```python
from build123d import *

# Parameters (mm, degrees)
SKETCH2_R          = 1.35
CUT_EXTRUDE1_DEPTH = 64.835726674
SKETCH4_R          = 25
CUT_EXTRUDE2_DEPTH = 64.835726674


with BuildPart() as part:
    # Sketch1 → Revolve1 (revolve)
    with BuildSketch(Plane.XY, mode=Mode.PRIVATE) as revolve1_sk:
        with BuildLine():
            Line((-42.5, 0), (0, 0))
            Line((0, 0), (0, 5))
            Line((0, 5), (-45, 5))
            Line((-45, 5), (-45, 2.5))
            ThreePointArc((-45, 2.5), (-43.232233047, 1.767766953), (-42.5, 0))
        make_face()
    revolve(revolve1_sk.sketch.rotate(Axis((0, 0, 0), (0, 1, 0)), 270), axis=Axis((0, 0, 0), (0, 1, 0)))

    # Sketch2 → Cut-Extrude1 (cut, through all)
    with BuildSketch(Plane(origin=(0, 5, 0), x_dir=(1, 0, 0), z_dir=(0, 1, 0))):
        with Locations(Location((0, 32.5, 0), (0, 0, 270))):
            Circle(SKETCH2_R)
        with Locations(Location((22.980970389, 22.980970389, 0), (0, 0, 270))):
            Circle(SKETCH2_R)
        with Locations(Location((32.5, 0, 0), (0, 0, 270))):
            Circle(SKETCH2_R)
        with Locations(Location((22.980970389, -22.980970389, 0), (0, 0, 270))):
            Circle(SKETCH2_R)
        with Locations(Location((0, -32.5, 0), (0, 0, 270))):
            Circle(SKETCH2_R)
        with Locations(Location((-22.980970389, -22.980970389, 0), (0, 0, 270))):
            Circle(SKETCH2_R)
        with Locations(Location((-32.5, 0, 0), (0, 0, 270))):
            Circle(SKETCH2_R)
        with Locations(Location((-22.980970389, 22.980970389, 0), (0, 0, 270))):
            Circle(SKETCH2_R)
    extrude(amount=-CUT_EXTRUDE1_DEPTH, mode=Mode.SUBTRACT)

    # Sketch4 → Cut-Extrude2 (cut, through all)
    with BuildSketch(Plane(origin=(0, 5, 0), x_dir=(1, 0, 0), z_dir=(0, 1, 0))):
        with Locations(Location((0, 0, 0), (0, 0, 270))):
            Circle(SKETCH4_R)
    extrude(amount=-CUT_EXTRUDE2_DEPTH, mode=Mode.SUBTRACT)


solid = part.part
```
Work out the finished part from the listing and answer in its coordinate system (mm). Coordinates: 2 decimals unless noted, no trailing zeros. Write each loop counter-clockwise with the first axis right and the second up, starting at its lowest first coordinate (ties: lowest second). Pieces come first, ordered by that corner, then holes.
Q1. A cutting plane is placed at A-A, the plane x = 0. Give the vertices of the cut face in (y, z), then the cut area to 3 significant figures.
Q2. Find the intervals of material crossed by line 1 (X direction, y = 3.9, z = 0); line 2 (X direction, y = 1.35, z = 0); line 3 (X direction, y = 0.3, z = 5), in increasing order.
Q3. This flat-tipped pin is pushed along its axis until it touches: pin 1 Ø2 at (x, y) = (-11, 4) entering from -Z. Where does it stop, or does it pass through?
Q4. A cutting plane is placed at B-B, the plane z = 0. Give the vertices of the cut face in (x, y).
Q5. Determine the mould class of faces 1 (the face through (19, 5, 19)), 2 (the face through (17.235, 3.732, -41.569)), 3 (the face through (31.18, 2.54, -0.29)) for opening direction X: released by +X, released by -X, zero draft, split by the parting line, or undercut.
Findings below:
1. outline: (0, -42.5) arc R2.5 cw to (2.5, -45) - (5, -45) - (5, -33.85) - (0, -33.85) - close; (0, -31.15) - (5, -31.15) - (5, -25) - (0, -25) - close; (0, 25) - (5, 25) - (5, 31.15) - (0, 31.15) - close; (0, 33.85) - (5, 33.85) - (5, 45) - (2.5, 45) arc R2.5 cw to (0, 42.5) - close
1. area: 163 mm2
2. line 1: x = -45 to -33.85, -31.15 to -25, 25 to 31.15, 33.85 to 45
2. line 2: x = -42.9 to -33.85, -31.15 to -25, 25 to 31.15, 33.85 to 42.9
2. line 3: x = -42.22 to -24.49, 24.49 to 42.22
3. pin 1: stops at z = -43.87
4. outline: (-45, 2.5) arc R2.5 cw to (-42.5, 0) - (-33.85, 0) - (-33.85, 5) - (-45, 5) - close; (-31.15, 0) - (-25, 0) - (-25, 5) - (-31.15, 5) - close; (25, 0) - (31.15, 0) - (31.15, 5) - (25, 5) - close; (33.85, 0) - (42.5, 0) arc R2.5 cw to (45, 2.5) - (45, 5) - (33.85, 5) - close
5. face 1: zero draft
5. face 2: split by the parting line
5. face 3: undercut
